Read the model definition and answer for the solid it produces. Units are mm, in the model's axes. Face numbers are marked on the shaded views. A direction names the side the tool comes from. Give positions to 0.01 mm unless a question says otherwise; leave off trailing zeros. Order: outer loops, then holes, each group sorted by start corner. A loop starts at its lowest first (then second) coordinate and runs counter-clockwise, first axis right, second up. Notation, with made-up numbers: (-16, 0.25) - (36, 0.25) arc R15 cw to (36, 19.25) - close; hole circle Ø2 at (39, 46). An arc over 180 degrees is marked (long way). Return JSON: item names as keys, results as strings.
```python
from build123d import *

# Parameters (mm, degrees)
SKETCH1_W           = 75.4
SKETCH1_H           = 9.4
BOSS_EXTRUDE1_DEPTH = 7
SKETCH2_R           = 0.75
SKETCH2_W           = 65.4
SKETCH2_H           = 3
CUT_EXTRUDE1_DEPTH  = 5
SKETCH3_W           = 2
SKETCH3_H           = 8
BOSS_EXTRUDE2_DEPTH = 5
BOSS_EXTRUDE3_DEPTH = 0.6


with BuildPart() as part:
    # Sketch1 → Boss-Extrude1 (new body)
    with BuildSketch(Plane.XY):
        Rectangle(SKETCH1_W, SKETCH1_H)
    extrude(amount=BOSS_EXTRUDE1_DEPTH)

    # Sketch2 → Cut-Extrude1 (cut)
    with BuildSketch(Plane.XY.offset(7)):
        with Locations((-35.5, 0)):
            Circle(SKETCH2_R)
        with Locations((35.5, 0)):
            Circle(SKETCH2_R)
        Rectangle(SKETCH2_W, SKETCH2_H)
    extrude(amount=-CUT_EXTRUDE1_DEPTH, mode=Mode.SUBTRACT)

    # Sketch3 → Boss-Extrude2 (add)
    with BuildSketch(Plane(origin=(0, 0, 0), x_dir=(-1, 0, 0), z_dir=(0, 0, -1))):
        with Locations((-36.7, 0)):
            Rectangle(SKETCH3_W, SKETCH3_H)
        with Locations((36.7, 0)):
            Rectangle(SKETCH3_W, SKETCH3_H)
    extrude(amount=BOSS_EXTRUDE2_DEPTH)

    # Sketch4 → Boss-Extrude3 (add, symmetric)
    with BuildSketch(Plane(origin=(0, 0, 0), x_dir=(1, 0, 0), z_dir=(0, 1, 0))):
        Polygon((10.169323516, 0), (15.169323516, 0), (15.169323516, -12), (14.669323516, -12), (14.669323516, -22), (10.669323516, -22), (10.669323516, -12), (10.169323516, -12), align=None)
    extrude(amount=BOSS_EXTRUDE3_DEPTH, both=True)


solid = part.part
```
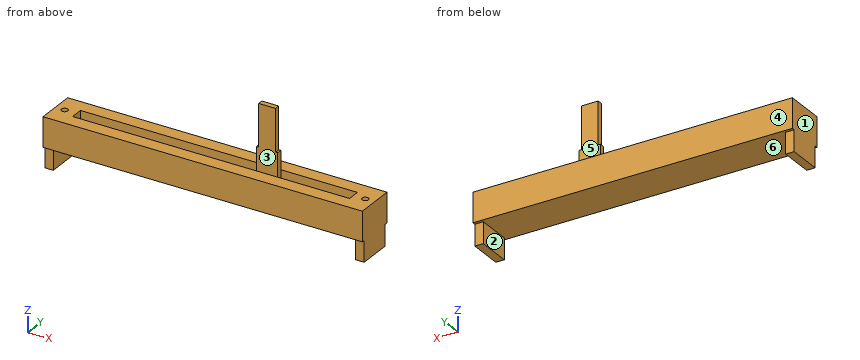
Q1. For the marked faces 1, 2 and 3, determine the directions among +Z, -Z, +X, -X, +Y, -Y from which every point of the face is accessible in a straight line to the end or side of a thin tool.
Values:
{"face 1": "+Z, -Z, -X, +Y, -Y", "face 2": "-Z, +Y, -Y", "face 3": "+Z"}
Q2. Given pin 1 (1.5 mm diameter, centred on x = 12.5, z = 11, fed in from -Y); pin 2 (3 mm diameter, centred on y = 0, z = 19.5, fed in from +X); pin 3 (3 mm diameter, centred on x = 8, y = -3.5, fed in from +Z), each flat-ended and moving along its own axis, determine where each tip first touches the part or whether it passes through.
Values:
{"pin 1": "stops at y = -0.6", "pin 2": "stops at x = 14.67", "pin 3": "stops at z = 7"}
Q3. A cutting plane is placed at C-C (y = 2.5). Write down the section's boundary in (x, z), and give its area (3 significant figures).
Values:
{"outline": "(-37.7, -5) - (-35.7, -5) - (-35.7, 0) - (35.7, 0) - (35.7, -5) - (37.7, -5) - (37.7, 7) - (-37.7, 7) - close", "area": "548 mm²"}
Q4. Determine the mould class of the marked faces 4, 5 and 6 for opening direction Y: released by +Y, released by -Y, zero draft, split by the parting line, or undercut.
Values:
{"face 4": "released by +Y", "face 5": "undercut", "face 6": "zero draft"}
Q5. A cutting plane is placed at B-B (x = 24.5). Write down the section's boundary in (y, z), and give its area (3 significant figures).
Values:
{"outline": "(-4.7, 0) - (4.7, 0) - (4.7, 7) - (1.5, 7) - (1.5, 2) - (-1.5, 2) - (-1.5, 7) - (-4.7, 7) - close", "area": "50.8 mm²"}
Q6. A cutting plane is placed at A-A (z = 5.5). Write down the section's boundary in (x, y).
Values:
{"outline": "(-37.7, -4.7) - (37.7, -4.7) - (37.7, 4.7) - (-37.7, 4.7) - close; (10.17, -0.6) - (15.17, -0.6) - (15.17, 0.6) - (10.17, 0.6) - close; hole circle Ø1.5 at (-35.5, 0); hole (-32.7, -1.5) - (32.7, -1.5) - (32.7, 1.5) - (-32.7, 1.5) - close; hole circle Ø1.5 at (35.5, 0)"}
Q7. A cutting plane is placed at D-D (z = 11.25). Write down the section's boundary in (x, y).
Values:
{"outline": "(10.17, -0.6) - (15.17, -0.6) - (15.17, 0.6) - (10.17, 0.6) - close"}
Q8. Consider L1, parallel to Y at x = -35.5, z = 3.6; L2, parallel to Y at x = 13, z = 3.5; L3, parallel to Y at x = -23, z = 2.5. Determine where each line is inside the solid, lowest interval first.
Values:
{"L1": "y = -4.7 to -0.75, 0.75 to 4.7", "L2": "y = -4.7 to -1.5, -0.6 to 0.6, 1.5 to 4.7", "L3": "y = -4.7 to -1.5, 1.5 to 4.7"}
